Geometry check sheet. Reference: the model listing, model coordinates, mm. A direction names the side the tool comes from. Round coordinates to 2 decimals unless told otherwise and drop trailing zeros. Write each loop counter-clockwise with the first axis right and the second up, starting at its lowest first coordinate (ties: lowest second). Pieces come first, ordered by that corner, then holes.
Item 1: Draft check along X on faces 3 (the face through (-1, -24, 2)), 4 (the face through (47.4, 23.43, 1.61)), 5 (the face through (24, 13, 2)). Enter one of: pulls with the +X half, pulls with the -X half, needs draft (parallel to the pull), parting line crosses it, or undercut.
Item 2: Cross-section at B-B (x = -24). Enter the section's corners in (y, z) (3 decimals), then the cut area to 3 significant figures.
Item 3: Cross-section at A-A (y = 0). Enter the section's corners in (x, z) (3 decimals).
Item 4: Cross-section at C-C (z = 1.35). State how many separate pieces and enclosed holes the cut face has, then the cut area to 3 significant figures.
Item 5: Depth check by flat-ended pin: P1, Ø4.5, axis at x = -8, y = 16, coming from the +Z side (3 decimals); P2, Ø20, axis at x = -24, y = 0, coming from the -Z side. Enter the tip coordinate at first touch or a pass-through.
Item 6: Cross-section at D-D (y = 19). Enter the section's corners in (x, z) (3 decimals), then the cut area to 3 significant figures.
Item 7: Scan lines: probe 1 along Y at (x, z) = (24, 1.8); probe 2 along X at (y, z) = (4, 0.7); probe 3 along Y at (x, z) = (-40, 1.4). Record each from-to range of solid material in increasing order.
Item 8: Access from +Z, -Z, +X, -X, +Y, -Y to the whole of each face (thin tool, end or side, straight path). Record for faces 1 (the face through (15.623, -14.961, 1.565)), 2 (the face through (-1, 24, 2)).
from build123d import *

# Parameters (mm, degrees)
SKETCH1_W           = 96
SKETCH1_H           = 48
SKETCH1_R           = 2.05
SKETCH1_R_2         = 11
BOSS_EXTRUDE1_DEPTH = 3.175
FILLET1_R           = 2


with BuildPart() as part:
    # Sketch1 → Boss-Extrude1 (new body)
    with BuildSketch(Plane.XY):
        Rectangle(SKETCH1_W, SKETCH1_H)
        with Locations((-40, 16)):
            Circle(SKETCH1_R, mode=Mode.SUBTRACT)
        with Locations((-8, 16)):
            Circle(SKETCH1_R, mode=Mode.SUBTRACT)
        with Locations((-8, -16)):
            Circle(SKETCH1_R, mode=Mode.SUBTRACT)
        with Locations((-40, -16)):
            Circle(SKETCH1_R, mode=Mode.SUBTRACT)
        with Locations((-24, 0)):
            Circle(SKETCH1_R_2, mode=Mode.SUBTRACT)
        with Locations(Location((8, 16, 0), (0, 0, 180))):
            Circle(SKETCH1_R, mode=Mode.SUBTRACT)
        with Locations(Location((8, -16, 0), (0, 0, 180))):
            Circle(SKETCH1_R, mode=Mode.SUBTRACT)
        with Locations(Location((40, -16, 0), (0, 0, 180))):
            Circle(SKETCH1_R, mode=Mode.SUBTRACT)
        with Locations(Location((24, 0, 0), (0, 0, 180))):
            Circle(SKETCH1_R_2, mode=Mode.SUBTRACT)
        with Locations(Location((40, 16, 0), (0, 0, 180))):
            Circle(SKETCH1_R, mode=Mode.SUBTRACT)
        Polygon((-38.544929421, 20.05), (-30, 13), (-18, 13), (-9.455070579, 20.05), align=None, mode=Mode.SUBTRACT)
        Polygon((-18, -13), (-9.455070579, -20.05), (-38.544929421, -20.05), (-30, -13), align=None, mode=Mode.SUBTRACT)
        Polygon((-11, -6), (-11, 6), (-4, 14.484327085), (4, 14.484327085), (11, 6), (11, -6), (4, -14.484327085), (-4, -14.484327085), align=None, mode=Mode.SUBTRACT)
        Polygon((30, -13), (18, -13), (9.455070579, -20.05), (38.544929421, -20.05), align=None, mode=Mode.SUBTRACT)
        Polygon((37, -6), (37, 6), (44, 14.484327085), (44, -14.484327085), align=None, mode=Mode.SUBTRACT)
        Polygon((18, 13), (9.455070579, 20.05), (38.544929421, 20.05), (30, 13), align=None, mode=Mode.SUBTRACT)
        Polygon((-44, -14.484327085), (-37, -6), (-37, 6), (-44, 14.484327085), align=None, mode=Mode.SUBTRACT)
    extrude(amount=BOSS_EXTRUDE1_DEPTH)

    # Fillet1
    fillet1_edges = [part.edges().sort_by_distance(p)[0] for p in [
        (38.544929421, -20.05, 1.5875),
        (30, -13, 1.5875),
        (18, -13, 1.5875),
        (9.455070579, -20.05, 1.5875),
        (37, -6, 1.5875),
        (44, -14.484327085, 1.5875),
        (44, 14.484327085, 1.5875),
        (37, 6, 1.5875),
        (18, 13, 1.5875),
        (30, 13, 1.5875),
        (38.544929421, 20.05, 1.5875),
        (9.455070579, 20.05, 1.5875),
        (-9.455070579, 20.05, 1.5875),
        (-38.544929421, 20.05, 1.5875),
        (-30, 13, 1.5875),
        (-18, 13, 1.5875),
        (-11, -6, 1.5875),
        (-4, -14.484327085, 1.5875),
        (4, -14.484327085, 1.5875),
        (11, -6, 1.5875),
        (11, 6, 1.5875),
        (4, 14.484327085, 1.5875),
        (-4, 14.484327085, 1.5875),
        (-11, 6, 1.5875),
        (-37, -6, 1.5875),
        (-37, 6, 1.5875),
        (-44, 14.484327085, 1.5875),
        (-44, -14.484327085, 1.5875),
        (-48, 24, 1.5875),
        (48, 24, 1.5875),
        (48, -24, 1.5875),
        (-48, -24, 1.5875),
        (-18, -13, 1.5875),
        (-30, -13, 1.5875),
        (-38.544929421, -20.05, 1.5875),
        (-9.455070579, -20.05, 1.5875),
    ]]
    fillet(fillet1_edges, radius=FILLET1_R)


solid = part.part
Resolved:
1. face 3: needs draft
1. face 4: pulls with the +X half
1. face 5: undercut
2. outline: (-24, 0) - (-20.05, 0) - (-20.05, 3.175) - (-24, 3.175) - close; (-13, 0) - (-11, 0) - (-11, 3.175) - (-13, 3.175) - close; (11, 0) - (13, 0) - (13, 3.175) - (11, 3.175) - close; (20.05, 0) - (24, 0) - (24, 3.175) - (20.05, 3.175) - close
2. area: 37.8 mm2
3. outline: (-48, 0) - (-44, 0) - (-44, 3.175) - (-48, 3.175) - close; (-37, 0) - (-35, 0) - (-35, 3.175) - (-37, 3.175) - close; (-13, 0) - (-11, 0) - (-11, 3.175) - (-13, 3.175) - close; (11, 0) - (13, 0) - (13, 3.175) - (11, 3.175) - close; (35, 0) - (37, 0) - (37, 3.175) - (35, 3.175) - close; (44, 0) - (48, 0) - (48, 3.175) - (44, 3.175) - close
4. separate pieces: 1
4. enclosed holes: 17
4. area: 2,430 mm2
5. P1: stops at z = 3.175
5. P2: passes through
6. outline: (-48, 0) - (-34.738, 0) - (-34.738, 3.175) - (-48, 3.175) - close; (-13.262, 0) - (13.262, 0) - (13.262, 3.175) - (-13.262, 3.175) - close; (34.738, 0) - (48, 0) - (48, 3.175) - (34.738, 3.175) - close
6. area: 168 mm2
7. probe 1: y = -24 to -20.05, -13 to -11, 11 to 13, 20.05 to 24
7. probe 2: x = -48 to -44, -37 to -34.25, -13.75 to -11, 11 to 13.75, 34.25 to 37, 44 to 48
7. probe 3: y = -24 to -18.05, -13.95 to -9.64, 9.64 to 13.95, 18.05 to 24
8. face 1: +Z, -Z
8. face 2: +Z, -Z, +X, -X, +Y
